Geometry: final body of the model. Coordinates: model frame, mm. Coordinates: 2 decimals unless noted, no trailing zeros. Order: outer loops, then holes, each group sorted by start corner. A loop starts at its lowest first (then second) coordinate and runs counter-clockwise, first axis right, second up. Notation, with made-up numbers: (57.25, 57.25) - (114.25, 57.25) arc R30 ccw to (114.25, 92.25) - close; hole circle Ø6 at (72.25, -14). An arc over 180 degrees is marked (long way). Use a Markdown table: item, result. Add a question column.
Autodesk Inventor part; units mm, degrees
ref_plane "YZ Plane" through (0, 0, 0) normal (1, 0, 0) x (0, 1, 0)
ref_plane "XZ Plane" through (0, 0, 0) normal (0, 1, 0) x (-1, 0, 0)
ref_plane "XY Plane" through (0, 0, 0) normal (0, 0, 1) x (1, 0, 0)
sketch "Sketch1" plane through (0, 0, 0) normal (0, 1, 0) x (-1, 0, 0)
  line L0 (5, 22) -> (-5, 22)
  line L1 (-5, 22) -> (-5, -20)
  line L2 (-5, -20) -> (5, -20)
  line L3 (5, -20) -> (5, 22)
  line L4 (0, 0) -> (5, 1) construction
  line L5 (0, 0) -> (-5, 1) construction
  line L6 (0, 0) -> (0, 22) construction
  line L7 (0, 0) -> (0, -20) construction
  dimension "d28" = 5
  dimension "d29" = 5
  dimension "d30" = 20
  dimension "d31" = 22
extrude "Extrusion1" add sketch "Sketch1" along normal blind 10
sketch "Sketch4" plane through (0, 10, 0) normal (0, 1, 0) x (1, 0, 0)
  circle A0 centre (0, 0) radius 2
  line L0 (0, 2) -> (0, 5) construction
  line L1 (0, 5) -> (0, 7.25) construction
  circle A1 centre (0, 7.25) radius 2.25
  line L2 (0, 9.5) -> (0, 15) construction
  circle A2 centre (0, 15) radius 2.5
  line L3 (0, -2) -> (0, -7.75) construction
  circle A3 centre (0, -7.75) radius 2.75
  line L4 (0, -10.5) -> (0, -16.5) construction
  circle A4 centre (0, -16.5) radius 3
  dimension "d19" = 4.5
  dimension "d23" = 5.5
  dimension "d16" = 4
  dimension "d17" = 3
  dimension "d18" = 2.25
  dimension "d20" = 5.5
  dimension "d21" = 5
  dimension "d22" = 5.75
  dimension "d24" = 6
  dimension "d25" = 6
extrude "Extrusion2" cut sketch "Sketch4" against normal through all
sketch "Sketch6" plane through (0, 10, 0) normal (0, 1, 0) x (1, 0, 0)
  circle A0 centre (-3.5576, -20.41) radius 1
  point P0 (0, 0)
  dimension "d32" = 2
extrude "Extrusion3" add sketch "Sketch6" along normal blind 1
properties part number "M4 test"
1) Pin query (flat end, axial travel): pin 1 (5 mm diameter, centred on x = 0, z = 0, fed in from +Y). Return the tip coordinate at first contact, or that it passes through.
2) Draft query along Z for faces 1 (the face through (5, 5, 1)), 2 (the face through (1.21, 5.07, -9.147)), 3 (the face through (-3.7, 10.5, 21.4)). Return one class per face: pulls with the +Z half, pulls with the -Z half, needs draft (parallel to the pull), parting line crosses it, or undercut.
3) Section D-D (z = -7.25). Return loops of the section in (x, y).
4) Ray query, line 1 along Z through (x, y) = (0, 3.5); line 2 along X through (y, z) = (6.5, -7.25); line 3 along Y through (x, z) = (-3, -13). Return the intervals inside material, ascending.
5) Section A-A (z = 7.75). Return loops of the section in (x, y).
6) Section B-B (y = 4.25). Return loops of the section in (x, z), then the cut area to 3 significant figures.
7) Section C-C (x = 0). Return loops of the section in (y, z), then the cut area to 3 significant figures.
Values follow:
| question | item | result |
|---|---|---|
| 1 | pin 1 | stops at y = 10 |
| 2 | face 1 | needs draft |
| 2 | face 2 | undercut |
| 2 | face 3 | parting line crosses it |
| 3 | outline | (-5, 0) - (-2.25, 0) - (-2.25, 10) - (-5, 10) - close; (2.25, 0) - (5, 0) - (5, 10) - (2.25, 10) - close |
| 4 | line 1 | z = -20 to -17.5, -12.5 to -9.5, -5 to -2, 2 to 5, 10.5 to 13.5, 19.5 to 22 |
| 4 | line 2 | x = -5 to -2.25, 2.25 to 5 |
| 4 | line 3 | y = 0 to 10 |
| 5 | outline | (-5, 0) - (-2.75, 0) - (-2.75, 10) - (-5, 10) - close; (2.75, 0) - (5, 0) - (5, 10) - (2.75, 10) - close |
| 6 | outline | (-5, -20) - (5, -20) - (5, 22) - (-5, 22) - close; hole circle Ø6 at (0, 16.5); hole circle Ø5.5 at (0, 7.75); hole circle Ø5 at (0, -15); hole circle Ø4.5 at (0, -7.25); hole circle Ø4 at (0, 0) |
| 6 | area | 320 mm² |
| 7 | outline | (0, -20) - (10, -20) - (10, -17.5) - (0, -17.5) - close; (0, -12.5) - (10, -12.5) - (10, -9.5) - (0, -9.5) - close; (0, -5) - (10, -5) - (10, -2) - (0, -2) - close; (0, 2) - (10, 2) - (10, 5) - (0, 5) - close; (0, 10.5) - (10, 10.5) - (10, 13.5) - (0, 13.5) - close; (0, 19.5) - (10, 19.5) - (10, 22) - (0, 22) - close |
| 7 | area | 170 mm² |
